```python
from build123d import *
from build123d.topology import SkipClean

# Parameters (mm, degrees)
SKETCH1_R           = 15.75
BOSS_EXTRUDE1_DEPTH = 10
CUT_EXTRUDE1_DEPTH  = 10
BOSS_EXTRUDE2_START = 3
BOSS_EXTRUDE2_DEPTH = 3
CHAMFER1_SIZE       = 2


with BuildPart() as part:
    # Sketch1 → Boss-Extrude1 (new body)
    with BuildSketch(Plane(origin=(0, 0, 0), x_dir=(1, 0, 0), z_dir=(0, 1, 0))):
        with Locations(Location((0, 0, 0), (0, 0, 270))):
            Circle(SKETCH1_R)
    extrude(amount=BOSS_EXTRUDE1_DEPTH)

    # Sketch2 → Cut-Extrude1 (cut)
    with BuildSketch(Plane(origin=(0, 10, 0), x_dir=(1, 0, 0), z_dir=(0, 1, 0))):
        Polygon((4.25, 2.453738644), (0, 4.907477288), (-4.25, 2.453738644), (-4.25, -2.453738644), (0, -4.907477288), (4.25, -2.453738644), align=None)
    extrude(amount=-CUT_EXTRUDE1_DEPTH, mode=Mode.SUBTRACT)

    # Sketch3 → Boss-Extrude2 (add)
    with SkipClean():  # the faces are left unmerged after this step: merging them gives an invalid solid
        with BuildSketch(Plane.XZ.offset(BOSS_EXTRUDE2_START)):
            with BuildLine():
                Line((-14.660328147, -5.756498818), (-7.8, 0))
                Line((-7.8, 0), (-14.660328147, 5.756498818))
                ThreePointArc((-14.660328147, 5.756498818), (-15.75, 0), (-14.660328147, -5.756498818))
            make_face()
            with BuildLine():
                Line((-3.9, -6.75499815), (-12.315438286, -9.817967194))
                ThreePointArc((-12.315438286, -9.817967194), (-7.875, -13.63990011), (-2.34488986, -15.574466011))
                Line((-2.34488986, -15.574466011), (-3.9, -6.75499815))
            make_face()
            with BuildLine():
                Line((3.9, -6.75499815), (2.34488986, -15.574466011))
                ThreePointArc((2.34488986, -15.574466011), (7.875, -13.63990011), (12.315438286, -9.817967194))
                Line((12.315438286, -9.817967194), (3.9, -6.75499815))
            make_face()
            with BuildLine():
                Line((7.8, 0), (14.660328147, -5.756498818))
                ThreePointArc((14.660328147, -5.756498818), (15.475184463, -2.929362703), (15.75, 0))
                ThreePointArc((15.75, 0), (15.475184463, 2.929362703), (14.660328147, 5.756498818))
                Line((14.660328147, 5.756498818), (7.8, 0))
            make_face()
            with BuildLine():
                ThreePointArc((12.315438286, 9.817967194), (7.875, 13.63990011), (2.34488986, 15.574466011))
                Line((2.34488986, 15.574466011), (3.9, 6.75499815))
                Line((3.9, 6.75499815), (12.315438286, 9.817967194))
            make_face()
            with BuildLine():
                ThreePointArc((-2.34488986, 15.574466011), (-7.875, 13.63990011), (-12.315438286, 9.817967194))
                Line((-12.315438286, 9.817967194), (-3.9, 6.75499815))
                Line((-3.9, 6.75499815), (-2.34488986, 15.574466011))
            make_face()
        extrude(amount=-BOSS_EXTRUDE2_DEPTH)

    # Chamfer1
    chamfer1_edges = [part.edges().sort_by_distance(p)[0] for p in [
        (4.25, 10, 0),
        (2.125, 10, -3.680607966),
        (-2.125, 10, -3.680607966),
        (-4.25, 10, 0),
        (-2.125, 10, 3.680607966),
        (2.125, 10, 3.680607966),
        (0, 10, -15.75),
    ]]
    chamfer(chamfer1_edges, length=CHAMFER1_SIZE)


solid = part.part
```
CAD build for the part. Positions are in the model's coordinates, mm. A direction names the side the tool comes from. Round coordinates to 2 decimals unless told otherwise and drop trailing zeros. Loops run counter-clockwise (first coordinate to the right, second up) from the corner with the lowest first, then second, coordinate; pieces in that order, holes last. Notation, with made-up numbers: M 40,55.25 L 64,55.25 A28 cw 64,77.25 Z; hole C 40.5,-40 d10. An arc over 180 degrees is marked long. Return JSON: item names as keys, results as strings. Group by question number.
(1) Saw through at C-C, the plane y = 9. List the corners of the cut face in (x, z), and give its area (3 significant figures).
(2) Mould opens along Z. For faces 4 (the flat face through (11.182, -1.521, -2.838)), 5 (the flat face through (-13, -3, 0)), 6 (the flat face through (-2.155, 4.056, 3.663)) say: +Z half, -Z half, draft (parallel to the pull), parting line (faces both ways), or undercut.
(3) Tool access for faces 1 (the flat face through (-11.182, -1.521, 2.838)), 2 (the flat face through (-4.25, 4, 0)), 3 (the flat face through (-8.17, -1.52, 8.31)): list every direction of +Z, -Z, +X, -X, +Y, -Y with a clear straight run to the whole face (end or side of a thin tool).
(4) Wall check: probe 1 along Z at (x, y) = (12, -0.5); probe 2 along Y at (x, z) = (3, -8.5); probe 3 along X at (y, z) = (8, 1.5). Give the ranges that are in metal, low to high. Write a range as [from, to].
(5) Saw through at A-A, the plane y = -2. Give the number of separate pieces and of enclosed holes in the cut face, and give its area (3 significant figures).
(6) Saw through at B-B, the plane y = 3. List the corners of the cut face in (x, z), and give its area (3 significant figures).
(7) Drop flat-ended pins along their axis: P1, Ø3, axis at y = 2.5, z = 10, coming from the +X side; P2, Ø1, axis at x = -4.5, z = -2.5, coming from the -Y side; P3, Ø5, axis at y = 8.5, z = 5, coming from the +X side. Give the stop position or say it passes through.
Answer list:
{
 "1": {"outline": "C 0,0 d29.5; hole M -5.25,-3.03 L 0,-6.06 L 5.25,-3.03 L 5.25,3.03 L 0,6.06 L -5.25,3.03 Z", "area": "588 mm2"},
 "2": {"face 4": "undercut", "face 5": "draft", "face 6": "undercut"},
 "3": {"face 1": "-Y", "face 2": "+Y, -Y", "face 3": "-X, -Y"},
 "4": {"probe 1": "[-10.2, -9.7], [-3.52, 3.52], [9.7, 10.2]", "probe 2": "[0, 10]", "probe 3": "[-15.68, -4.25], [4.25, 15.68]"},
 "5": {"separate pieces": "6", "enclosed holes": "0", "area": "287 mm2"},
 "6": {"outline": "C 0,0 d31.5; hole M -4.25,-2.45 L 0,-4.91 L 4.25,-2.45 L 4.25,2.45 L 0,4.91 L -4.25,2.45 Z", "area": "717 mm2"},
 "7": {"P1": "x = 13.26", "P2": "y = 0", "P3": "x = 15.54"}
}
